For this review, take the finished solid that the model builds, in its own axes (mm). A direction names the side the tool comes from. Coordinates: 2 decimals unless noted, no trailing zeros. Loops run counter-clockwise (first coordinate to the right, second up) from the corner with the lowest first, then second, coordinate; pieces in that order, holes last. Notation, with made-up numbers: (35.25, -13.75) -> (71.25, -13.75) arc R20 ccw to (71.25, -6.75) -> close; hole circle Ø9 at (46, 9). An arc over 180 degrees is marked (long way). Use a Markdown table: item, result.
from build123d import *

# Parameters (mm, degrees)
BOSS_EXTRUDE1_DEPTH  = 1.5875
FILLET2_R            = 1.778
M4_CLEARANCE_HOLE2_D = 4.5


with BuildPart() as part:
    # Sketch1 → Boss-Extrude1 (new body)
    with BuildSketch(Plane.XY):
        with BuildLine():
            Line((-3.078924099, 16.382133449), (-3.078924099, -25.617866551))
            Line((-3.078924099, -25.617866551), (2.159951047, -25.617866551))
            Line((2.159951047, -25.617866551), (7.399260817, -25.617866551))
            Line((7.399260817, -25.617866551), (7.399260817, 4.381445812))
            Line((7.399260817, 4.381445812), (7.399260817, 19.381445781))
            Line((7.399260817, 19.381445781), (13.018541309, 37.070554481))
            ThreePointArc((13.018541309, 37.070554481), (3.802061978, 31.484715671), (-6.508003397, 34.622810382))
            Line((-6.508003397, 34.622810382), (-3.078924099, 16.382133449))
        make_face()
    extrude(amount=BOSS_EXTRUDE1_DEPTH)

    # Fillet2
    fillet2_edges = [part.edges().sort_by_distance(p)[0] for p in [
        (-3.078924099, -25.617866551, 0.79375),
        (-6.508003397, 34.622810382, 0.79375),
        (13.018541309, 37.070554481, 0.79375),
        (7.399260817, -25.617866551, 0.79375),
    ]]
    fillet(fillet2_edges, radius=FILLET2_R)

    # M4 Clearance Hole2 (through all)
    with Locations(Plane.XY.offset(1.5875)):
        with Locations((2.160168359, 5.103784263), (2.160168359, -15.895866551)):
            Hole(M4_CLEARANCE_HOLE2_D / 2)


solid = part.part
(1) Take a section at D-D on y = -8.5. Write out the cut boundary in (x, z), plus the area to 3 significant figures.
Found:
| item | result |
|---|---|
| outline | (-3.08, 0) -> (7.4, 0) -> (7.4, 1.59) -> (-3.08, 1.59) -> close |
| area | 16.6 mm^2 |
(2) For pin 1 Ø0.5 at (y, z) = (-5, 0.5) entering from +X; pin 2 Ø2.5 at (x, y) = (2.16, 5.1) entering from -Z; pin 3 Ø8 at (x, y) = (-4, -6) entering from -Z, all flat-tipped, find the tip position at first contact; note any pin that passes through.
Found:
| item | result |
|---|---|
| pin 1 | stops at x = 7.4 |
| pin 2 | passes through |
| pin 3 | stops at z = 0 |
(3) Take a section at B-B on z = 0.4. Write out the cut boundary in (x, y).
Found:
| item | result |
|---|---|
| outline | (-5.75, 30.6) -> (-3.08, 16.38) -> (-3.08, -23.84) arc R1.78 ccw to (-1.3, -25.62) -> (5.62, -25.62) arc R1.78 ccw to (7.4, -23.84) -> (7.4, 19.38) -> (11.06, 30.91) arc R1.78 ccw to (8.51, 33.01) arc R13.21 cw to (-3.27, 32.55) arc R1.78 ccw to start; hole circle Ø4.5 at (2.16, -15.9); hole circle Ø4.5 at (2.16, 5.1) |
(4) Take a section at C-C on x = 0.5. Write out the cut boundary in (y, z), plus the area to 3 significant figures.
Found:
| item | result |
|---|---|
| outline | (-25.62, 0) -> (-17.41, 0) -> (-17.41, 1.59) -> (-25.62, 1.59) -> close; (-14.38, 0) -> (3.59, 0) -> (3.59, 1.59) -> (-14.38, 1.59) -> close; (6.62, 0) -> (31.49, 0) -> (31.49, 1.59) -> (6.62, 1.59) -> close |
| area | 81.0 mm^2 |
(5) Take a section at A-A on y = -17.5. Write out the cut boundary in (x, z).
Found:
| item | result |
|---|---|
| outline | (-3.08, 0) -> (0.58, 0) -> (0.58, 1.59) -> (-3.08, 1.59) -> close; (3.74, 0) -> (7.4, 0) -> (7.4, 1.59) -> (3.74, 1.59) -> close |
(6) For faces 4 (the face through (7.399, -3, 1)), 5 (the face through (2.453, -13.665, 0.783)), 6 (the face through (-3.079, -3, 1)), list the 3-axis set-ups (+Z, -Z, +X, -X, +Y, -Y) from which the entire face can be reached by the end or side of a thin tool; tool diameter is ignored.
Found:
| item | result |
|---|---|
| face 4 | +Z, -Z, +X, -Y |
| face 5 | +Z, -Z |
| face 6 | +Z, -Z, -X, -Y |
(7) Mouldability with a two-part tool opening along X and no side actions: class faces 1 (the face through (3, 11, 0)), 2 (the face through (2.759, 31.396, 0.783)), 3 (the face through (-4.434, 23.591, 0.783)) as pulls with the +X half, pulls with the -X half, needs draft (parallel to the pull), parting line crosses it, or undercut.
Found:
| item | result |
|---|---|
| face 1 | needs draft |
| face 2 | undercut |
| face 3 | pulls with the -X half |
(8) For line 1 along Y through (x, z) = (3.5, 0.45); line 2 along Y through (x, z) = (1.25, 1.2); line 3 along X through (y, z) = (-21, 0.25), list the stretches that pass through material, from the lowest coordinate up.
Found:
| item | result |
|---|---|
| line 1 | y = -25.62 to -17.7, -14.09 to 3.3, 6.91 to 31.45 |
| line 2 | y = -25.62 to -17.95, -13.84 to 3.05, 7.16 to 31.41 |
| line 3 | x = -3.08 to 7.4 |
